Work out the finished part from the listing and answer in its coordinate system (mm). Face numbers are marked on the shaded views. A direction names the side the tool comes from. Coordinates: 2 decimals unless noted, no trailing zeros. Loops run counter-clockwise (first coordinate to the right, second up) from the corner with the lowest first, then second, coordinate; pieces in that order, holes last. Notation, with made-up numbers: (1, -33.75) -> (48, -33.75) arc R20 ccw to (48, -13.75) -> close; hole circle Ø6 at (-6, 33.5). An arc over 180 degrees is marked (long way). Answer as CSV lines item,"result".
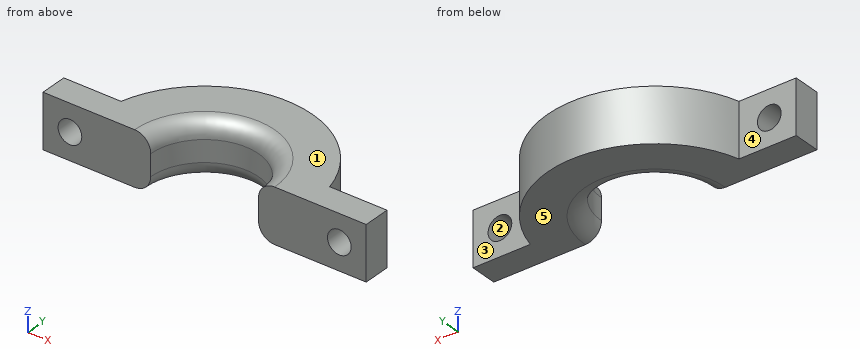
```python
from build123d import *

# Parameters (mm, degrees)
REVOLVE1_ANGLE      = 180
SKETCH2_R           = 2.2
BOSS_EXTRUDE1_DEPTH = 5


with BuildPart() as part:
    # Sketch1 → Revolve1 (revolve)
    with BuildSketch(Plane(origin=(0, 0, 0), x_dir=(1, 0, 0), z_dir=(0, 1, 0))):
        with BuildLine():
            Line((-20, 0), (-13, 0))
            ThreePointArc((-13, 0), (-10.878679656, 0.878679656), (-10, 3))
            Line((-10, 3), (-10, 7))
            ThreePointArc((-10, 7), (-10.878679656, 9.121320344), (-13, 10))
            Line((-13, 10), (-20, 10))
            Line((-20, 10), (-20, 0))
        make_face()
    revolve(axis=Axis((0, 0, 0), (0, 0, -1)), revolution_arc=REVOLVE1_ANGLE)

    # Sketch2 → Boss-Extrude1 (add)
    # profile 1 of 2: a face of its own
    with BuildSketch(Plane.XZ):
        Polygon((-20, 0), (-30, 0), (-30, -10), (-20, -10), (-16.5, -10), (-16.5, 0), align=None)
        with Locations(Location((-25, -5, 0), (0, 0, 270))):
            Circle(SKETCH2_R, mode=Mode.SUBTRACT)
    # profile 2 of 2: a face of its own
    with BuildSketch(Plane.XZ):
        Polygon((20, 0), (30, 0), (30, -10), (20, -10), (16.5, -10), (16.5, 0), align=None)
        with Locations(Location((25, -5, 0), (0, 0, 270))):
            Circle(SKETCH2_R, mode=Mode.SUBTRACT)
    extrude(amount=-BOSS_EXTRUDE1_DEPTH)


solid = part.part
```
(1) Consider line 1 along X through (y, z) = (1.4, -5); line 2 along X through (y, z) = (2.25, -5); line 3 along Y through (x, z) = (-22.5, -3.75). Determine where each line is inside the solid, lowest interval first.
Computed values:
line 1,"-30 to -27.2, -22.8 to -9.9, 9.9 to 22.8, 27.2 to 30"
line 2,"-30 to -27.2, -22.8 to -9.74, 9.74 to 22.8, 27.2 to 30"
line 3,"0 to 5"
(2) A cutting plane is placed at A-A, the plane x = 25. Write down the section's boundary in (y, z).
Computed values:
outline,"(0, -10) -> (5, -10) -> (5, -7.2) -> (0, -7.2) -> close; (0, -2.8) -> (5, -2.8) -> (5, 0) -> (0, 0) -> close"
(3) A cutting plane is placed at C-C, the plane y = 3. Count the separate pieces of the cut face and the enclosed holes in it, and give its area (3 significant figures).
Computed values:
separate pieces,"2"
enclosed holes,"2"
area,"371 mm2"
(4) For a pull along Z with two mould halves and no side action, classify the marked faces 1, 2 and 3 as pulls with the +Z half, pulls with the -Z half, needs draft (parallel to the pull), parting line crosses it, or undercut.
Computed values:
face 1,"pulls with the +Z half"
face 2,"undercut"
face 3,"needs draft"
(5) Flat-ended cylindrical pins translate along their axes: pin 1 Ø3 at (y, z) = (16, -2) entering from -X (3 decimals); pin 2 Ø3 at (x, z) = (-25.5, -3.5) entering from +Y; pin 3 Ø4 at (y, z) = (18, -5) entering from -X. Find the tip coordinate at first contact, or state that the pin passes through.
Computed values:
pin 1,"x = -13.775"
pin 2,"y = 5"
pin 3,"x = -12"
(6) Which of the six approach directions +Z, -Z, +X, -X, +Y, -Y give full straight-line access (tool end or side, diameter ignored) to the marked faces 4 and 5?
Computed values:
face 4,"+Z, -Z, -X, +Y"
face 5,"-Z, +X, -X, +Y, -Y"
(7) A cutting plane is placed at D-D, the plane x = 0. Write down the section's boundary in (y, z).
Computed values:
outline,"(10, -7) arc R3 ccw to (13, -10) -> (20, -10) -> (20, 0) -> (13, 0) arc R3 ccw to (10, -3) -> close"
(8) A cutting plane is placed at B-B, the plane z = -5. Write down the section's boundary in (x, y), and give its area (3 significant figures).
Computed values:
outline,"(-30, 0) -> (-27.2, 0) -> (-27.2, 5) -> (-30, 5) -> close; (-22.8, 0) -> (-10, 0) arc R10 cw to (10, 0) -> (22.8, 0) -> (22.8, 5) -> (19.36, 5) arc R20 ccw to (-19.36, 5) -> (-22.8, 5) -> close; (27.2, 0) -> (30, 0) -> (30, 5) -> (27.2, 5) -> close"
area,"529 mm2"
